Check sheet for the modelled part. Datum: model origin and axes. Units: mm. A direction names the side the tool comes from. Round coordinates to 2 decimals unless told otherwise and drop trailing zeros. Put each result on its own line as item: value. Start each with the question number.
Item 1: Draft check along Z on faces 3 (the flat face through (161, -5, -115)), 4 (the flat face through (142, -5, 0)), 5 (the cylindrical face through (140.29, -2.46, -60.72)), 6 (the flat face through (138, -5, -150)). Enter one of: pulls with the +Z half, pulls with the -Z half, needs draft (parallel to the pull), parting line crosses it, or undercut.
Item 2: Gauge pin test, flat ends, axial feed: pin 1 Ø6 at (x, z) = (270, -112.92) entering from -Y; pin 2 Ø3 at (x, z) = (20, -60) entering from -Y (3 decimals); pin 3 Ø7.5 at (x, z) = (162, -74) entering from -Y. Record the tip position at first contact, or that the pin passes through.
Item 3: Material ranges on line 1 along X through (y, z) = (-8.95, -60); line 2 along Z through (x, y) = (10, -7.75); line 3 along Z through (x, y) = (270, -1.75), recorded low to high.
Item 4: Tool access check on faces 1 (the flat face through (0, -5, -74)), 2 (the cylindrical face through (158.88, -7.54, -69.82)). Record the directions out of +Z, -Z, +X, -X, +Y, -Y that give a thin tool (end or side, any length) a straight path to the whole face; none if there is none.
from build123d import *

# Parameters (mm, degrees)
BOSS_EXTRUDE1_DEPTH                      = 10
CBORE_FOR_M4_PAN_HEAD_SCREW1_D           = 4.8
CBORE_FOR_M4_PAN_HEAD_SCREW1_CBORE_D     = 9
CBORE_FOR_M4_PAN_HEAD_SCREW1_CBORE_DEPTH = 5
M3X0_5_TAPPED_HOLE1_D                    = 2.5
CBORE_FOR_M3_PAN_HEAD_SCREW1_D           = 3.6
CBORE_FOR_M3_PAN_HEAD_SCREW1_CBORE_D     = 7
CBORE_FOR_M3_PAN_HEAD_SCREW1_CBORE_DEPTH = 5


with BuildPart() as part:
    # Sketch1 → Boss-Extrude1 (new body)
    with BuildSketch(Plane(origin=(0, 0, 0), x_dir=(1, 0, 0), z_dir=(0, 1, 0))):
        Polygon((0, 145), (5, 150), (275, 150), (280, 145), (280, 5), (275, 0), (5, 0), (0, 5), align=None)
    extrude(amount=-BOSS_EXTRUDE1_DEPTH)

    # CBORE for M4 Pan Head Screw1 (through all)
    with Locations(Plane(origin=(0, -10, 0), x_dir=(-1, 0, 0), z_dir=(0, -1, 0))):
        with Locations((-138, 60), (-20, 60)):
            CounterBoreHole(CBORE_FOR_M4_PAN_HEAD_SCREW1_D / 2, CBORE_FOR_M4_PAN_HEAD_SCREW1_CBORE_D / 2, CBORE_FOR_M4_PAN_HEAD_SCREW1_CBORE_DEPTH)

    # M3x0.5 Tapped Hole1 (through all)
    with Locations(Plane(origin=(0, -10, 0), x_dir=(-1, 0, 0), z_dir=(0, -1, 0))):
        with Locations((-10, 10), (-10, 140), (-270, 140), (-270, 10)):
            Hole(M3X0_5_TAPPED_HOLE1_D / 2)

    # CBORE for M3 Pan Head Screw1 (through all)
    with Locations(Plane(origin=(0, -10, 0), x_dir=(-1, 0, 0), z_dir=(0, -1, 0))):
        with Locations((-160.5, 112.922675535), (-160.5, 72.922675535), (-270, 112.922675535), (-270, 72.922675535)):
            CounterBoreHole(CBORE_FOR_M3_PAN_HEAD_SCREW1_D / 2, CBORE_FOR_M3_PAN_HEAD_SCREW1_CBORE_D / 2, CBORE_FOR_M3_PAN_HEAD_SCREW1_CBORE_DEPTH)


solid = part.part
Check result:
1. face 3: undercut
1. face 4: pulls with the +Z half
1. face 5: undercut
1. face 6: pulls with the -Z half
2. pin 1: y = -5
2. pin 2: through
2. pin 3: y = -10
3. line 1: 0 to 15.5, 24.5 to 133.5, 142.5 to 280
3. line 2: -150 to -141.25, -138.75 to -11.25, -8.75 to 0
3. line 3: -150 to -141.25, -138.75 to -114.72, -111.12 to -74.72, -71.12 to -11.25, -8.75 to 0
4. face 1: +Z, -Z, -X, +Y, -Y
4. face 2: -Y
